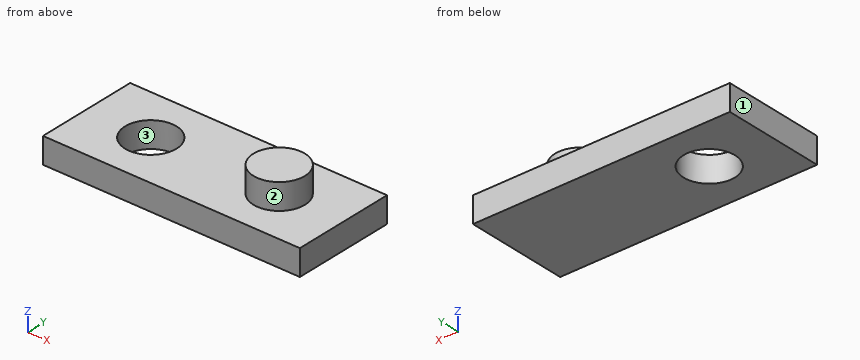
from build123d import *

# Parameters (mm, degrees)
F0_W     = 63.5
F0_H     = 25.4
F1_DEPTH = 6.35
F2_R     = 6.35
F3_DEPTH = 6.351
F4_R     = 6.35
F5_DEPTH = 6.35


with BuildPart() as f1:
    # F0 (on Top) → F1 (new body)
    with BuildSketch(Plane.XY):
        Rectangle(F0_W, F0_H)
    extrude(amount=F1_DEPTH)

    # F2 (on face) → F3 (cut, through all)
    with BuildSketch(Plane.XY.offset(6.35)):
        with Locations((-15.875, 0)):
            Circle(F2_R)
    extrude(amount=-F3_DEPTH, mode=Mode.SUBTRACT)

    # F4 (on face) → F5 (join)
    with BuildSketch(Plane.XY.offset(6.35)):
        with Locations((15.875, 0)):
            Circle(F4_R)
    extrude(amount=F5_DEPTH)


solid = f1.part
Can you work these out from the model? Positions are in its coordinate system, mm. Face numbers are marked on the shaded views. Round coordinates to 2 decimals unless told otherwise and drop trailing zeros. Write each loop counter-clockwise with the first axis right and the second up, starting at its lowest first coordinate (ties: lowest second). Pieces come first, ordered by that corner, then holes. Notation, with made-up numbers: (-30.75, -14.75) -> (-3.75, -14.75) arc R27 cw to (-3.75, 13.25) -> close; hole circle Ø1 at (23, 79.5). An arc over 180 degrees is marked (long way). One line per question, with ' | ' between items. Start each with the question number.
1) Suppose I cut it at C-C on x = -21. Write out the boundary of the cut face in (y, z), then the cut area to 3 significant figures.
2) I'm going to push flat-ended pins straight in: P1, Ø1.5, axis at y = 0, z = 8, coming from the +X side (3 decimals); P2, Ø12.5, axis at x = -4.5, y = -6, coming from the +Z side. Where does each tip first touch, or does it pass through?
3) Suppose I cut it at B-B on z = 5.5. Write out the boundary of the cut face in (x, y) (3 decimals), then the cut area to 3 significant figures.
4) Suppose I cut it at A-A on y = 0. Write out the boundary of the cut face in (x, z) (3 decimals).
5) If we mould it in two halves opening along Y, with no side actions, what happens to the marked faces 1, 2 and 3? For each: released by +Y, released by -Y, zero draft, split by the parting line, or undercut.
6) Suppose I cut it at D-D on x = 18. Write out the boundary of the cut face in (y, z).
7) I need wall thicknesses on line 1 (Z direction, x = -17, y = 11.5); line 2 (X direction, y = 5, z = 6); line 3 (X direction, y = -0.75, z = 1.5). Which ranges of each line are inside material? Lowest first, please. Write a range as [from, to].
Return value:
1) outline: (-12.7, 0) -> (-3.75, 0) -> (-3.75, 6.35) -> (-12.7, 6.35) -> close; (3.75, 0) -> (12.7, 0) -> (12.7, 6.35) -> (3.75, 6.35) -> close | area: 114 mm2
2) P1: stops at x = 22.225 | P2: stops at z = 6.35
3) outline: (-31.75, -12.7) -> (31.75, -12.7) -> (31.75, 12.7) -> (-31.75, 12.7) -> close; hole circle Ø12.7 at (-15.875, 0) | area: 1,490 mm2
4) outline: (-31.75, 0) -> (-22.225, 0) -> (-22.225, 6.35) -> (-31.75, 6.35) -> close; (-9.525, 0) -> (31.75, 0) -> (31.75, 6.35) -> (22.225, 6.35) -> (22.225, 12.7) -> (9.525, 12.7) -> (9.525, 6.35) -> (-9.525, 6.35) -> close
5) face 1: zero draft | face 2: split by the parting line | face 3: undercut
6) outline: (-12.7, 0) -> (12.7, 0) -> (12.7, 6.35) -> (5.98, 6.35) -> (5.98, 12.7) -> (-5.98, 12.7) -> (-5.98, 6.35) -> (-12.7, 6.35) -> close
7) line 1: z = [0, 6.35] | line 2: x = [-31.75, -19.79], [-11.96, 31.75] | line 3: x = [-31.75, -22.18], [-9.57, 31.75]
